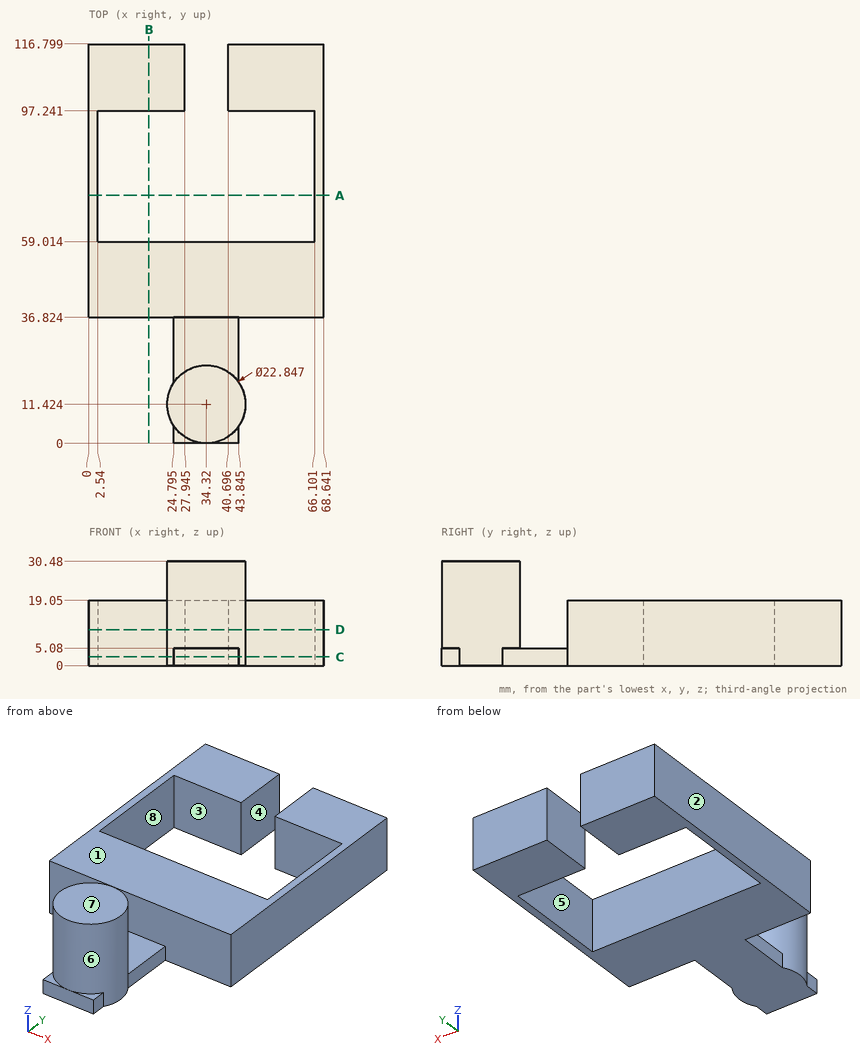
Geometry: see drawing. Coordinates: mm, zero at the bounding-box minimum. A direction names the side the tool comes from. Coordinates: 2 decimals unless noted, no trailing zeros. Loops run counter-clockwise (first coordinate to the right, second up) from the corner with the lowest first, then second, coordinate; pieces in that order, holes last. Notation, with made-up numbers: (16.25, 55) -> (34.25, 55) arc R9 ccw to (34.25, 62) -> close; hole circle Ø2 at (45, 17). An arc over 180 degrees is marked (long way). Write item = value, one per line. Start each with the question number.
Item 1: Mould query, pull axis X, two halves, no side actions, for the marked faces 5, 6, 7 and 8. Classes: pulls with the +X half, pulls with the -X half, needs draft (parallel to the pull), parting line crosses it, or undercut.
Item 2: Cut plane C-C, the plane z = 2.5. Return loops of the section in (x, y) (1 decimal).
Item 3: Cut plane B-B, the plane x = 17.5. Return loops of the section in (y, z).
Item 4: First-contact query: P1, Ø3, axis at x = 25.5, y = 50, coming from the +Z side; P2, Ø2, axis at x = 21, z = 21.5, coming from the +Y side; P3, Ø5.5, axis at x = 15, z = 10, coming from the -Y side; P4, Ø15, axis at y = 103.5, z = 13.5, coming from the -X side. Flat tips, straight axial feed; report the tip coordinate or a pass-through.
Item 5: Cut plane D-D, the plane z = 10.5. Return loops of the section in (x, y) (1 decimal), plus the area to 3 significant figures.
Item 6: Cut plane A-A, the plane y = 72.5. Return loops of the section in (x, z).
Item 7: Reachability of the marked faces 1, 2, 3 and 4 from +Z, -Z, +X, -X, +Y, -Y: full face, straight path, thin tool, end or side. Return the list, or none.
Item 8: Material intervals for line 1 (Y direction, x = 7, z = 6); line 2 (X direction, y = 96, z = 7); line 3 (X direction, y = 111, z = 5.5) (1 decimal), sorted ascending.
Ans:
q1.face_5 = undercut
q1.face_6 = parting line crosses it
q1.face_7 = needs draft
q1.face_8 = undercut
q2.outline = (0, 36.8) -> (24.8, 36.8) -> (24.8, 17.7) arc R11.4 ccw to (24.8, 5.1) -> (24.8, 0) -> (43.8, 0) -> (43.8, 5.1) arc R11.4 ccw to (43.8, 17.7) -> (43.8, 36.8) -> (68.6, 36.8) -> (68.6, 116.8) -> (40.7, 116.8) -> (40.7, 97.2) -> (66.1, 97.2) -> (66.1, 59) -> (2.5, 59) -> (2.5, 97.2) -> (27.9, 97.2) -> (27.9, 116.8) -> (0, 116.8) -> close
q3.outline = (36.82, 0) -> (59.01, 0) -> (59.01, 19.05) -> (36.82, 19.05) -> close; (97.24, 0) -> (116.8, 0) -> (116.8, 19.05) -> (97.24, 19.05) -> close
q4.P1 = 19.05
q4.P2 = through
q4.P3 = 36.82
q4.P4 = 0
q5.outline = (0, 36.8) -> (68.6, 36.8) -> (68.6, 116.8) -> (40.7, 116.8) -> (40.7, 97.2) -> (66.1, 97.2) -> (66.1, 59) -> (2.5, 59) -> (2.5, 97.2) -> (27.9, 97.2) -> (27.9, 116.8) -> (0, 116.8) -> close; circle Ø22.8 at (34.3, 11.4)
q5.area = 3,220 mm²
q6.outline = (0, 0) -> (2.54, 0) -> (2.54, 19.05) -> (0, 19.05) -> close; (66.1, 0) -> (68.64, 0) -> (68.64, 19.05) -> (66.1, 19.05) -> close
q7.face_1 = +Z, +X, -X, +Y
q7.face_2 = +Z, -Z, -X, +Y, -Y
q7.face_3 = +Z, -Z
q7.face_4 = +Z, -Z, +Y
q8.line_1 = 36.82 to 59.01, 97.24 to 116.8
q8.line_2 = 0 to 2.54, 66.1 to 68.64
q8.line_3 = 0 to 27.9, 40.7 to 68.6
